Geometry check sheet. Reference: the model listing, model coordinates, mm. Face numbers are marked on the shaded views. A direction names the side the tool comes from. Give positions to 0.01 mm unless a question says otherwise; leave off trailing zeros. Write each loop counter-clockwise with the first axis right and the second up, starting at its lowest first coordinate (ties: lowest second). Pieces come first, ordered by that corner, then holes. Notation, with made-up numbers: (-4, 79.5) - (20, 79.5) arc R22 cw to (20, 112.5) - close; hole circle Ø6 at (-35.75, 67). An arc over 180 degrees is marked (long way). Use a Markdown table: item, result.
```python
from build123d import *

# Parameters (mm, degrees)
F0_R     = 1
F1_DEPTH = 3.5
F2_DEPTH = 2
F3_DEPTH = 2


# Not quite as in the source:
# - a feature names something its author has since deleted; it is built from what else it names


with BuildPart() as f1:
    # F0 (on Top) → F1 (new body)
    with BuildSketch(Plane.XY):
        with Locations((-2.3999998812, 1.8953582125)):
            Circle(F0_R)
    extrude(amount=F1_DEPTH)



with BuildPart() as f1b:
    # F0 (on Top) → F1, piece 2 (new body)
    with BuildSketch(Plane.XY):
        with Locations((-2.3991598333, -2.1004185153)):
            Circle(F0_R)
    extrude(amount=F1_DEPTH)


with BuildPart() as f1_1:
    add(f1.part)

    add(f1b.part)  # F2 merges F1b
    # F0 (on Top) → F2 (join)
    with BuildSketch(Plane.XY):
        with BuildLine():
            ThreePointArc((-2.4958517574, -0.1027572147), (-3.8471556634, -0.7208141967), (-4.3991598333, -2.1004185153))
            ThreePointArc((-4.3991598333, -2.1004185153), (-2.3991598333, -4.1004185153), (-0.3991598333, -2.1004185153))
            ThreePointArc((-0.3991598333, -2.1004185153), (-0.9511640032, -0.7208141967), (-2.3024679093, -0.1027572147))
            ThreePointArc((-2.3024679093, -0.1027572147), (-2.3991598333, -0.1050959142), (-2.4958517574, -0.1027572147))
        make_face()
        with Locations((-2.3991598333, -2.1004185153)):
            Circle(F0_R, mode=Mode.SUBTRACT)
        with BuildLine():
            ThreePointArc((-2.3024679093, -0.1027572147), (-0.9511640032, -0.7208141967), (-0.3991598333, -2.1004185153))
            Line((-0.3991598333, -2.1004185153), (-0.3991598333, 1.8949040858))
            ThreePointArc((-0.3991598333, 1.8949040858), (-0.9511640032, 0.5152997672), (-2.3024679093, -0.1027572147))
        make_face()
        with BuildLine():
            ThreePointArc((-4.3991598333, 1.8949040858), (-3.8471556634, 0.5152997672), (-2.4958517574, -0.1027572147))
            ThreePointArc((-2.4958517574, -0.1027572147), (-2.3991598333, -0.1004185153), (-2.3024679093, -0.1027572147))
            ThreePointArc((-2.3024679093, -0.1027572147), (-0.9511640032, 0.5152997672), (-0.3991598333, 1.8949040858))
            ThreePointArc((-0.3991598333, 1.8949040858), (-2.3991598333, 3.8949040858), (-4.3991598333, 1.8949040858))
        make_face()
        with Locations((-2.3999998812, 1.8953582125)):
            Circle(F0_R, mode=Mode.SUBTRACT)
        with BuildLine():
            ThreePointArc((-2.3024679093, -0.1027572147), (-2.3991598333, -0.1004185153), (-2.4958517574, -0.1027572147))
            ThreePointArc((-2.4958517574, -0.1027572147), (-2.3991598333, -0.1050959142), (-2.3024679093, -0.1027572147))
        make_face()
    extrude(amount=F2_DEPTH)

    # F0 (on Top) → F3 (join)
    with BuildSketch(Plane.XY):
        with BuildLine():
            Line((-4.3991598333, 1.8949040858), (-4.3991598333, -2.1004185153))
            ThreePointArc((-4.3991598333, -2.1004185153), (-3.8471556634, -0.7208141967), (-2.4958517574, -0.1027572147))
            ThreePointArc((-2.4958517574, -0.1027572147), (-3.8471556634, 0.5152997672), (-4.3991598333, 1.8949040858))
        make_face()
    extrude(amount=F3_DEPTH)


solid = f1_1.part
```
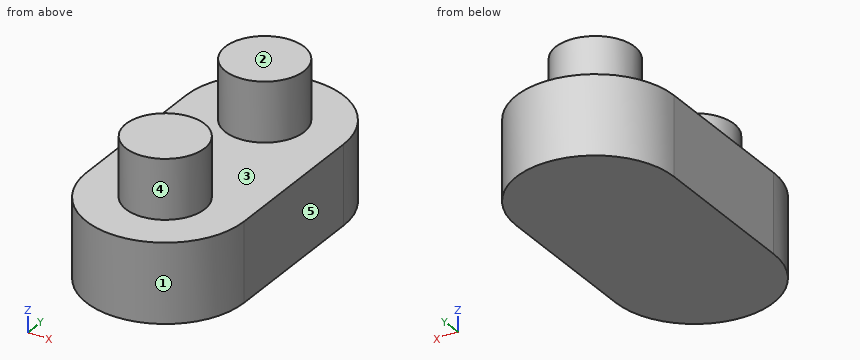
1) Section check B-B on y = -2. Record the boundary of the cut face in (x, z), then the cut area to 3 significant figures.
Working result:
| item | result |
|---|---|
| outline | (-4.4, 0) - (-0.4, 0) - (-0.4, 2) - (-1.4, 2) - (-1.4, 3.5) - (-3.39, 3.5) - (-3.39, 2) - (-4.4, 2) - close |
| area | 11.0 mm² |
2) Mould release check, pull along Y, two halves, no side actions. Record for the marked faces 1, 2 and 3: pulls with the +Y half, pulls with the -Y half, needs draft (parallel to the pull), parting line crosses it, or undercut.
Working result:
| item | result |
|---|---|
| face 1 | pulls with the -Y half |
| face 2 | needs draft |
| face 3 | undercut |
3) Set-up check for the marked faces 4 and 5: record each of +Z, -Z, +X, -X, +Y, -Y from which the full face is reachable in a straight line by a thin tool's end or side.
Working result:
| item | result |
|---|---|
| face 4 | +Z |
| face 5 | +Z, -Z, +X, +Y, -Y |
4) Section check D-D on x = -1.7. Record the boundary of the cut face in (y, z), then the cut area to 3 significant figures.
Working result:
| item | result |
|---|---|
| outline | (-3.97, 0) - (3.77, 0) - (3.77, 2) - (2.61, 2) - (2.61, 3.5) - (1.18, 3.5) - (1.18, 2) - (-1.39, 2) - (-1.39, 3.5) - (-2.82, 3.5) - (-2.82, 2) - (-3.97, 2) - close |
| area | 19.8 mm² |
5) Material ranges on L1, parallel to Z at x = -4, y = 2.5; L2, parallel to Y at x = -3.2, z = 2.9; L3, parallel to Y at x = -2.5, z = 2.35, recorded low to high. Write a range as from..to.
Working result:
| item | result |
|---|---|
| L1 | z = 0..2 |
| L2 | y = -2.7..-1.5, 1.3..2.5 |
| L3 | y = -3.1..-1.11, 0.9..2.89 |
6) Section check A-A on x = -2.4. Record the boundary of the cut face in (y, z), then the cut area to 3 significant figures.
Working result:
| item | result |
|---|---|
| outline | (-4.1, 0) - (3.89, 0) - (3.89, 2) - (2.9, 2) - (2.9, 3.5) - (0.9, 3.5) - (0.9, 2) - (-1.1, 2) - (-1.1, 3.5) - (-3.1, 3.5) - (-3.1, 2) - (-4.1, 2) - close |
| area | 22.0 mm² |
7) Section check C-C on z = 2.2. Record the boundary of the cut face in (x, y).
Working result:
| item | result |
|---|---|
| outline | circle Ø2 at (-2.4, -2.1); circle Ø2 at (-2.4, 1.9) |
